Verification items for the finished model (mm, model axes). Face numbers are marked on the shaded views. A direction names the side the tool comes from. Give positions to 0.01 mm unless a question says otherwise; leave off trailing zeros. Write each loop counter-clockwise with the first axis right and the second up, starting at its lowest first coordinate (ties: lowest second). Pieces come first, ordered by that corner, then holes. Notation, with made-up numbers: (11.5, 58) - (22.5, 58) arc R23 cw to (22.5, 91) - close; hole circle Ø9 at (24, -3.5). An arc over 180 degrees is marked (long way). Answer as a JSON object with one key per item and string values. Group by question number.
Item 1: Go/stop test with flat-tipped pins: pin 1 (10 mm diameter, centred on x = -18.5, z = -8.5, fed in from +Y); pin 2 (10 mm diameter, centred on x = -31.5, z = 8, fed in from -Y); pin 3 (1 mm diameter, centred on y = -38, z = -4, fed in from +X); pin 4 (19.5 mm diameter, centred on x = 0, y = 0, fed in from +Z). Record where each tip stops, or that it passes through.
Item 2: Tool access check on the marked faces 1 and 2. Record the directions out of +Z, -Z, +X, -X, +Y, -Y that give a thin tool (end or side, any length) a straight path to the whole face; none if there is none.
Item 3: Draft check along Y on the marked faces 3, 4 and 5. Enter one of: +Y half, -Y half, draft (parallel to the pull), parting line (faces both ways), or undercut.
Item 4: Scan lines: line 1 along Y through (x, z) = (0, 0.75); line 2 along Y through (x, z) = (-2, 0.5); line 3 along X through (y, z) = (1, -6.5). Record each from-to range of solid material in increasing order. Write a range as [from, to].
Item 5: Sectioned sample at C-C, the plane z = 2. Record the boundary of the cut face in (x, y).
Item 6: Sectioned sample at D-D, the plane z = -5.5. Record the boundary of the cut face in (x, y).
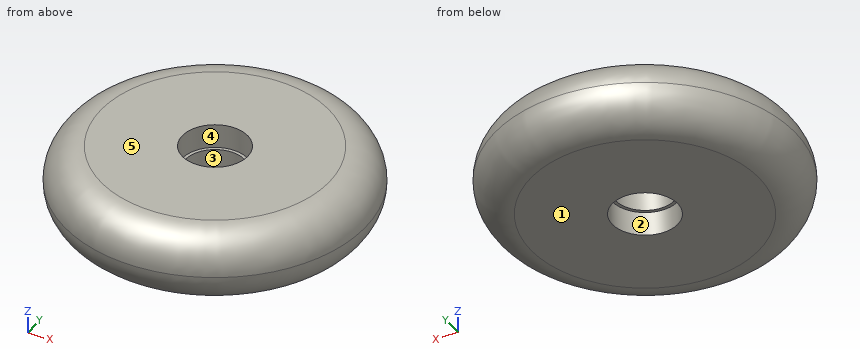
Autodesk Inventor part; units mm, degrees
ref_plane "YZ Plane" through (0, 0, 0) normal (1, 0, 0) x (0, 1, 0)
ref_plane "XZ Plane" through (0, 0, 0) normal (0, 1, 0) x (-1, 0, 0)
ref_plane "XY Plane" through (0, 0, 0) normal (0, 0, 1) x (1, 0, 0)
sketch "Sketch1" plane through (0, 0, 0) normal (0, 0, 1) x (1, 0, 0)
  circle A0 centre (0, 0) radius 50
  dimension "d0" = 100
extrude "Extrusion1" add sketch "Sketch1" along normal mid plane 24
fillet "Fillet1" radius 12 2 edges at (-50, 0, 12) (-50, 0, -12)
sketch "Sketch2" plane through (0, 0, 12) normal (0, 0, 1) x (1, 0, 0)
  point P0 (0, 0)
sketch "Sketch3" plane through (0, 0, 12) normal (0, 0, 1) x (1, 0, 0)
  circle A0 centre (0, 0) radius 10.9
  dimension "d4" = 21.8
extrude "Extrusion2" cut sketch "Sketch3" against normal through all
sketch "Sketch4" plane through (0, 0, 0) normal (0, 0, 1) x (1, 0, 0)
  circle A0 centre (0, 0) radius 9.8
  circle A1 centre (0, 0) radius 10.9
  circle A2 centre (0, 0) radius 10.9
  dimension "d7" = 19.6
extrude "Extrusion4" add sketch "Sketch4" along normal mid plane 8
properties part number "WHEEL" material "Rubber"
Geometry check:
{
 "1": {"pin 1": "y = 46.62", "pin 2": "y = -40.45", "pin 3": "x = 32.08", "pin 4": "through"},
 "2": {"face 1": "-Z, +X, -X, +Y, -Y", "face 2": "-Z"},
 "3": {"face 3": "undercut", "face 4": "undercut", "face 5": "draft"},
 "4": {"line 1": "[-49.98, -9.8], [9.8, 49.98]", "line 2": "[-49.95, -9.59], [9.59, 49.95]", "line 3": "[-48.08, -10.85], [10.85, 48.08]"},
 "5": {"outline": "circle Ø99.66 at (0, 0); hole circle Ø19.6 at (0, 0)"},
 "6": {"outline": "circle Ø97.33 at (0, 0); hole circle Ø21.8 at (0, 0)"}
}
